For this review, take the finished solid that the model builds, in its own axes (mm). A direction names the side the tool comes from. Round coordinates to 2 decimals unless told otherwise and drop trailing zeros. Write each loop counter-clockwise with the first axis right and the second up, starting at its lowest first coordinate (ties: lowest second). Pieces come first, ordered by that corner, then holes. Notation, with made-up numbers: M 36.5,54.25 L 64.5,54.25 A16 cw 64.5,58.25 Z; hole C 54,16.25 d9. An arc over 180 degrees is marked long. One line per question, with ' | ' between items.
```python
from build123d import *

# Parameters (mm, degrees)
SKETCH1_R               = 8.5
SKETCH1_R_2             = 7.55
BOSS_EXTRUDE1_DEPTH     = 5
SKETCH2_R               = 8.5
SKETCH2_R_2             = 1.1
BOSS_EXTRUDE2_DEPTH     = 2
SKETCH3_R               = 3.5
SKETCH3_R_2             = 1.5
BOSS_EXTRUDE3_DEPTH     = 15
CUT_EXTRUDE1_DEPTH      = 20.222382787
CUT_EXTRUDE1_DEPTH_BACK = 20.222382787
SKETCH3_3_R             = 1.1
SKETCH4_R               = 1.6
SKETCH4_R_2             = 1.1
BOSS_EXTRUDE4_DEPTH     = 5
BOSS_EXTRUDE5_START     = -0.3
SKETCH5_R               = 1.1
BOSS_EXTRUDE5_DEPTH     = 0.3
FILLET1_R               = 1


with BuildPart() as part:
    # Sketch1 → Boss-Extrude1 (new body)
    with BuildSketch(Plane.XY):
        Circle(SKETCH1_R)
        Circle(SKETCH1_R_2, mode=Mode.SUBTRACT)
    extrude(amount=BOSS_EXTRUDE1_DEPTH)

    # Sketch2 → Boss-Extrude2 (add)
    with BuildSketch(Plane.XY.offset(5)):
        Circle(SKETCH2_R)
        Circle(SKETCH2_R_2, mode=Mode.SUBTRACT)
    extrude(amount=BOSS_EXTRUDE2_DEPTH)

    # Sketch3 → Boss-Extrude3 (add)
    with BuildSketch(Plane.XY.offset(7)):
        Circle(SKETCH3_R)
        Circle(SKETCH3_R_2, mode=Mode.SUBTRACT)
    extrude(amount=BOSS_EXTRUDE3_DEPTH)

    # Sketch3<3> → Cut-Extrude1 (cut, two sides: drawn at the far end of the back side and taken through both)
    with BuildSketch(Plane.XY.offset(7).offset(-CUT_EXTRUDE1_DEPTH_BACK)):
        with Locations((-5.5, 0)):
            Circle(SKETCH3_3_R)
        with Locations((5.5, 0)):
            Circle(SKETCH3_3_R)
    extrude(amount=CUT_EXTRUDE1_DEPTH + CUT_EXTRUDE1_DEPTH_BACK, mode=Mode.SUBTRACT)

    # Sketch4 → Boss-Extrude4 (add)
    # profile 1 of 3: a face of its own
    with BuildSketch(Plane(origin=(0, 0, 5), x_dir=(-1, 0, 0), z_dir=(0, 0, -1))):
        with Locations(Location((5.5, 0, 0), (0, 0, 180))):
            Circle(SKETCH4_R)
        with Locations(Location((5.5, 0, 0), (0, 0, 180))):
            Circle(SKETCH4_R_2, mode=Mode.SUBTRACT)
    # profile 2 of 3: a face of its own
    with BuildSketch(Plane(origin=(0, 0, 5), x_dir=(-1, 0, 0), z_dir=(0, 0, -1))):
        with Locations(Location((0, 0, 0), (0, 0, 180))):
            Circle(SKETCH4_R)
        with Locations(Location((0, 0, 0), (0, 0, 180))):
            Circle(SKETCH4_R_2, mode=Mode.SUBTRACT)
    # profile 3 of 3: a face of its own
    with BuildSketch(Plane(origin=(0, 0, 5), x_dir=(-1, 0, 0), z_dir=(0, 0, -1))):
        with Locations(Location((-5.5, 0, 0), (0, 0, 180))):
            Circle(SKETCH4_R)
        with Locations(Location((-5.5, 0, 0), (0, 0, 180))):
            Circle(SKETCH4_R_2, mode=Mode.SUBTRACT)
    extrude(amount=BOSS_EXTRUDE4_DEPTH)

    # Sketch5 → Boss-Extrude5 (add)
    with BuildSketch(Plane(origin=(0, 0, 5), x_dir=(-1, 0, 0), z_dir=(0, 0, -1)).offset(BOSS_EXTRUDE5_START)):
        with Locations(Location((5.5, 0, 0), (0, 0, 180))):
            Circle(SKETCH5_R)
        with Locations(Location((-5.5, 0, 0), (0, 0, 180))):
            Circle(SKETCH5_R)
        Circle(SKETCH5_R)
    extrude(amount=BOSS_EXTRUDE5_DEPTH)

    # Fillet1
    fillet1_edges = [part.edges().sort_by_distance(p)[0] for p in [
        (-8.5, 0, 7),
        (-3.5, 0, 22),
    ]]
    fillet(fillet1_edges, radius=FILLET1_R)


solid = part.part
```
Item 1: Take a section at B-B (z = 8). Write out the cut boundary in (x, y), then the cut area to 3 significant figures.
Results:
outline: C 0,0 d7; hole C 0,0 d3 | area: 31.4 mm2
Item 2: Take a section at A-A (z = 4.5). Write out the cut boundary in (x, y), then the cut area to 3 significant figures.
Results:
outline: C 0,0 d17; C -5.5,0 d3.2; C 0,0 d3.2; C 5.5,0 d3.2; hole C 0,0 d15.1; hole C -5.5,0 d2.2; hole C 0,0 d2.2; hole C 5.5,0 d2.2 | area: 60.6 mm2
Item 3: Mouldability with a two-part tool opening along X and no side actions: class faces 1 (the face through (-1.8, -3.2, 7)), 2 (the face through (4.57, 7.167, 2.958)), 3 (the face through (-4.02, 0.61, 2.54)) as +X half, -X half, draft (parallel to the pull), parting line (faces both ways), or undercut.
Results:
face 1: draft | face 2: parting line | face 3: undercut
Item 4: Machinability: for faces 4 (the face through (5, 0, 5)), 5 (the face through (-1.5, 0.07, 14.4)), 6 (the face through (0, 8, 0)), which of the approach directions +Z, -Z, +X, -X, +Y, -Y give a long, thin tool a straight path to every point of the face, cutting with its end or side? Answer none if there is none.
Results:
face 4: -Z | face 5: +Z | face 6: -Z, +X, -X, +Y, -Y
Item 5: Insertion check: pin 1 Ø2.5 at (x, y) = (5.5, -0.5) entering from +Z; pin 2 Ø2 at (x, y) = (5.5, 0) entering from -Z; pin 3 Ø5 at (y, z) = (1, 9) entering from +X; pin 4 Ø4 at (x, y) = (0, 0) entering from -Z. Each pin has a flat end and moves straight along its axis. Give the tip position at first contact, or say it passes through.
Results:
pin 1: z = 7 | pin 2: z = 5 | pin 3: x = 8.33 | pin 4: z = 0
Item 6: To check wall thickness, follow line 1 along Z through (x, y) = (5.25, 3.5); line 2 along Z through (x, y) = (0.5, 0); line 3 along Y through (x, z) = (-4.75, 6.25). State the ranges of each line that lie inside material, in increasing order. Write a range as from..to.
Results:
line 1: 5..7 | line 2: 5..5.3 | line 3: -7.01..-0.8, 0.8..7.01
